Read the model definition and answer for the solid it produces. Units are mm, in the model's axes. A direction names the side the tool comes from. Coordinates: 2 decimals unless noted, no trailing zeros. Loops run counter-clockwise (first coordinate to the right, second up) from the corner with the lowest first, then second, coordinate; pieces in that order, holes last. Notation, with made-up numbers: M 19,-28 L 66,-28 A20 ccw 66,-1 Z; hole C 86.25,83 d9. An arc over 180 degrees is marked long. One line per item, written item: value. Start each with the question number.
1. The part is cut by section C-C (y = 39.5). Write down the section's boundary in (x, z), then the cut area to 3 significant figures.
2. The part is cut by section D-D (z = 1.55). State how many separate pieces and enclosed holes the cut face has, then the cut area to 3 significant figures.
3. The part is cut by section A-A (x = 0). Write down the section's boundary in (y, z), then the cut area to 3 significant figures.
4. For faces 5 (the face through (0, 60, 1)), 6 (the face through (-70.5, -25.59, 1.52)), determine the directions among +Z, -Z, +X, -X, +Y, -Y from which every point of the face is accessible in a straight line to the end or side of a thin tool.
5. Determine the mould class of faces 1 (the face through (34.93, -60.5, 1.48)), 2 (the face through (-6, 61, 3)), 3 (the face through (38.939, 67.585, 1.521)), 4 (the face through (-73.32, 26.61, 1.52)) for opening direction Y: +Y half, -Y half, draft (parallel to the pull), parting line (faces both ways), or undercut.
6. Consider probe 1 along Y at (x, z) = (-36, 2.35); probe 2 along Y at (x, z) = (34, 2.8); probe 3 along X at (y, z) = (25.5, 2.8). Determine where each line is inside the solid, lowest interval first.
7. The part is cut by section B-B (y = 0). Write down the section's boundary in (x, z), then the cut area to 3 significant figures.
8. Flat-ended cylindrical pins translate along their axes: pin 1 (1.5 mm diameter, centred on x = 16, z = 2.5, fed in from +Y); pin 2 (1.5 mm diameter, centred on y = 65, z = 1.5, fed in from -X); pin 3 (1.5 mm diameter, centred on x = 58, z = 2, fed in from +Y). Find the tip coordinate at first contact, or state that the pin passes through.
```python
from build123d import *

# Parameters (mm, degrees)
P_IDAT_VYSUNUT_M1_DEPTH  = 3
SKICA3_W                 = 12
SKICA3_H                 = 3
SKICA3_W_2               = 3
SKICA3_H_2               = 10
ODEBRAT_VYSUNUT_M1_DEPTH = 3
SKICA4_W                 = 48
SKICA4_H                 = 3.5
ODEBRAT_VYSUNUT_M3_DEPTH = 3


with BuildPart() as part:
    # Skica1 → Přidat vysunutím1 (new body)
    with BuildSketch(Plane.XY):
        with BuildLine():
            Line((-40, -69.282032303), (-30, -51.961524227))
            ThreePointArc((-30, -51.961524227), (0, 60), (30, -51.961524227))
            Line((30, -51.961524227), (40, -69.282032303))
            ThreePointArc((40, -69.282032303), (0, 80), (-40, -69.282032303))
        make_face()
    extrude(amount=P_IDAT_VYSUNUT_M1_DEPTH)

    # Skica3 → Odebrat vysunutím1 (cut)
    with BuildSketch(Plane.XY.offset(3)):
        Polygon((-43.330127019, 65.049981495), (-34.669872981, 70.049981495), (-33.169872981, 67.451905284), (-41.830127019, 62.451905284), align=None)
        with Locations((0, 64.5)):
            Rectangle(SKICA3_W, SKICA3_H)
        Polygon((-18.468596623, 75.946763847), (-8.620519093, 77.683245623), (-8.09957456, 74.728822364), (-17.94765209, 72.992340588), align=None)
        Polygon((8.620519093, 77.683245623), (18.468596623, 75.946763847), (17.94765209, 72.992340588), (8.09957456, 74.728822364), align=None)
        Polygon((34.669872981, 70.049981495), (43.330127019, 65.049981495), (41.830127019, 62.451905284), (33.169872981, 67.451905284), align=None)
        Polygon((56.537528515, 53.967655771), (62.965404612, 46.30721134), (60.667271282, 44.378848511), (54.239395185, 52.039292942), align=None)
        Polygon((71.585923705, 31.376034283), (75.006125138, 21.979108075), (72.187047276, 20.953047646), (68.766845842, 30.349973853), align=None)
        with Locations((76.5, 0)):
            Rectangle(SKICA3_W_2, SKICA3_H_2)
        Polygon((75.006125138, -21.979108075), (71.585923705, -31.376034283), (68.766845842, -30.349973853), (72.187047276, -20.953047645), align=None)
        Polygon((62.965404612, -46.30721134), (56.537528515, -53.967655771), (54.239395186, -52.039292942), (60.667271282, -44.378848511), align=None)
        Polygon((-56.537528515, -53.967655771), (-62.965404612, -46.30721134), (-60.667271282, -44.378848511), (-54.239395185, -52.039292942), align=None)
        Polygon((-71.585923705, -31.376034283), (-75.006125138, -21.979108075), (-72.187047276, -20.953047645), (-68.766845842, -30.349973853), align=None)
        with Locations((-76.5, 0)):
            Rectangle(SKICA3_W_2, SKICA3_H_2)
        Polygon((-75.006125138, 21.979108075), (-71.585923705, 31.376034283), (-68.766845842, 30.349973853), (-72.187047276, 20.953047645), align=None)
        Polygon((-62.965404612, 46.30721134), (-56.537528515, 53.967655771), (-54.239395185, 52.039292942), (-60.667271282, 44.378848511), align=None)
    extrude(amount=-ODEBRAT_VYSUNUT_M1_DEPTH, mode=Mode.SUBTRACT)

    # Skica4 → Odebrat vysunutím3 (cut)
    with BuildSketch(Plane(origin=(0, 0, 0), x_dir=(-1, 0, 0), z_dir=(0, 0, -1))):
        with Locations((0, 54.56)):
            Rectangle(SKICA4_W, SKICA4_H)
    extrude(amount=-ODEBRAT_VYSUNUT_M3_DEPTH, mode=Mode.SUBTRACT)


solid = part.part
```
Answer block:
1. outline: M -69.57,0 L -45.16,0 L -45.16,3 L -69.57,3 Z; M 45.16,0 L 69.57,0 L 69.57,3 L 45.16,3 Z
1. area: 146 mm2
2. separate pieces: 1
2. enclosed holes: 15
2. area: 6,870 mm2
3. outline: M 60,0 L 63,0 L 63,3 L 60,3 Z; M 66,0 L 80,0 L 80,3 L 66,3 Z
3. area: 51.0 mm2
4. face 5: +Z, -Z, -Y
4. face 6: +Z, -Z
5. face 1: -Y half
5. face 2: draft
5. face 3: undercut
5. face 4: undercut
6. probe 1: y = -62.35 to -48, 48 to 65.82, 69.28 to 71.44
6. probe 2: y = -58.89 to -49.44, 49.44 to 66.97, 68.89 to 72.42
6. probe 3: x = -75.83 to -73.72, -70.53 to -54.31, 54.31 to 70.53, 73.72 to 75.83
7. outline: M -80,0 L -78,0 L -78,3 L -80,3 Z; M -75,0 L -60,0 L -60,3 L -75,3 Z; M 60,0 L 75,0 L 75,3 L 60,3 Z; M 78,0 L 80,0 L 80,3 L 78,3 Z
7. area: 102 mm2
8. pin 1: stops at y = 78.53
8. pin 2: stops at x = -47.66
8. pin 3: stops at y = 55.88
